from build123d import *

# Parameters (mm, degrees)
ESQUISSE2_W             = 17
ESQUISSE2_H             = 22
BASE_DEPTH              = 42
ESQUISSE3_R             = 6
VIDE_CERCLE_DEPTH       = 2
ESQUISSE4_R             = 1
AXE_ROUE_DEPTH          = 8
ESQUISSE6_R             = 1.5
COTE_DEPTH              = 4
ESQUISSE7_W             = 10.5
ESQUISSE7_H             = 8
AJUSTE_COTE_DEPTH       = 4
ESQUISSE8_W             = 7
ESQUISSE8_H             = 1
BLOC_MOTEUR_DEPTH       = 31
VODE_START              = -15
VODE_MOTEUR_DEPTH       = 15
ESQUISSE11_R            = 1
SORTIE_AXE_MOTEUR_DEPTH = 1
VIS_MOTEUR_1_DEPTH      = 6
VIS_MOTEUR_2_DEPTH      = 2
ESQUISSE15_R            = 1
VIS_MOTEUR_3_DEPTH      = 1


with BuildPart() as part:
    # Esquisse2 → Base (new body)
    with BuildSketch(Plane(origin=(0, 0, 0), x_dir=(1, 0, 0), z_dir=(0, 1, 0))):
        with Locations((-30.697167752, 0)):
            Rectangle(ESQUISSE2_W, ESQUISSE2_H)
    extrude(amount=-BASE_DEPTH)

    # Esquisse3 → VIDE CERCLE (cut)
    with BuildSketch(Plane.ZY.offset(39.197167752)):
        with Locations((0, -8.724551396)):
            Circle(ESQUISSE3_R)
        with Locations(Location((0, -33.275448604, 0), (0, 0, 180))):
            Circle(ESQUISSE3_R)
    extrude(amount=-VIDE_CERCLE_DEPTH, mode=Mode.SUBTRACT)

    # Esquisse4 → AXE ROUE (add)
    with BuildSketch(Plane.ZY.offset(37.197167752)):
        with BuildLine():
            Line((1.785357107, -6.974551396), (-1.785357107, -6.974551396))
            ThreePointArc((-1.785357107, -6.974551396), (-2.5, -8.724551396), (-1.785357107, -10.474551396))
            Line((-1.785357107, -10.474551396), (1.785357107, -10.474551396))
            ThreePointArc((1.785357107, -10.474551396), (2.5, -8.724551396), (1.785357107, -6.974551396))
        make_face()
        with Locations((0, -8.724551396)):
            Circle(ESQUISSE4_R, mode=Mode.SUBTRACT)
    extrude(amount=AXE_ROUE_DEPTH)

    # Esquisse6 → COTE (add)
    with BuildSketch(Plane.XY.offset(11)):
        with BuildLine():
            Line((-19.697167752, -2), (-16.197167752, -2))
            ThreePointArc((-16.197167752, -2), (-15.490060971, -2.292893219), (-15.197167752, -3))
            Line((-15.197167752, -3), (-15.197167752, -9))
            ThreePointArc((-15.197167752, -9), (-15.490060971, -9.707106781), (-16.197167752, -10))
            Line((-16.197167752, -10), (-19.697167752, -10))
            ThreePointArc((-19.697167752, -10), (-20.395192088, -10.520394841), (-21.197167752, -10.859339966))
            Line((-21.197167752, -10.859339966), (-21.197167752, -42))
            Line((-21.197167752, -42), (-22.197167752, -42))
            Line((-22.197167752, -42), (-22.197167752, -49))
            ThreePointArc((-22.197167752, -49), (-22.490060971, -49.707106781), (-23.197167752, -50))
            Line((-23.197167752, -50), (-31.697167752, -50))
            ThreePointArc((-31.697167752, -50), (-32.404274533, -49.707106781), (-32.697167752, -49))
            Line((-32.697167752, -49), (-32.697167752, -42))
            Line((-32.697167752, -42), (-39.197167752, -42))
            Line((-39.197167752, -42), (-39.197167752, 0))
            Line((-39.197167752, 0), (-22.197167752, 0))
            Line((-22.197167752, 0), (-21.197167752, 0))
            Line((-21.197167752, 0), (-21.197167752, -1.140660034))
            ThreePointArc((-21.197167752, -1.140660034), (-20.395192088, -1.479605159), (-19.697167752, -2))
        make_face()
        with Locations((-19.697167752, -6)):
            Circle(ESQUISSE6_R, mode=Mode.SUBTRACT)
        with Locations((-28.697167752, -35)):
            Circle(ESQUISSE6_R, mode=Mode.SUBTRACT)
        with Locations((-28.697167752, -45)):
            Circle(ESQUISSE6_R, mode=Mode.SUBTRACT)
    cote = extrude(amount=COTE_DEPTH)

    # SYM COTE: COTE across plane
    add(cote.mirror(Plane.XY))

    # Esquisse7 → AJUSTE COTE (cut)
    with BuildSketch(Plane.XY.offset(-11)):
        with Locations((-27.447167752, -46)):
            Rectangle(ESQUISSE7_W, ESQUISSE7_H)
    extrude(amount=-AJUSTE_COTE_DEPTH, mode=Mode.SUBTRACT)

    # Esquisse8 → BLOC MOTEUR (add)
    with BuildSketch(Plane(origin=(-22.197167752, 0, 0), x_dir=(0, 0, -1), z_dir=(1, 0, 0))):
        with BuildLine():
            ThreePointArc((-5.878988008, -24), (-10.75, -33), (-5.878988008, -42))
            Line((-5.878988008, -42), (-3.5, -42))
            Line((-3.5, -42), (3.5, -42))
            Line((3.5, -42), (5.878988008, -42))
            ThreePointArc((5.878988008, -42), (10.75, -33), (5.878988008, -24))
            Line((5.878988008, -24), (3.5, -24))
            Line((3.5, -24), (-3.5, -24))
            Line((-3.5, -24), (-5.878988008, -24))
        make_face()
        with Locations((0, -42.5)):
            Rectangle(ESQUISSE8_W, ESQUISSE8_H)
        with Locations((0, -23.5)):
            Rectangle(ESQUISSE8_W, ESQUISSE8_H)
    extrude(amount=BLOC_MOTEUR_DEPTH)

    # Esquisse10 → VODE MOTEUR (cut)
    with BuildSketch(Plane(origin=(8.802832248, 0, 0), x_dir=(0, 0, -1), z_dir=(1, 0, 0)).offset(VODE_START)):
        with BuildLine():
            Line((-5.878988008, -24), (-3.5, -24))
            Line((-3.5, -24), (-3.5, -25))
            Line((-3.5, -25), (-5.573374202, -25))
            ThreePointArc((-5.573374202, -25), (-9.75, -33), (-5.573374202, -41))
            Line((-5.573374202, -41), (-3.5, -41))
            Line((-3.5, -41), (-3.5, -42))
            Line((-3.5, -42), (-5.878988008, -42))
            ThreePointArc((-5.878988008, -42), (-10.75, -33), (-5.878988008, -24))
        make_face()
        with BuildLine():
            Line((3.5, -24), (5.878988008, -24))
            ThreePointArc((5.878988008, -24), (10.75, -33), (5.878988008, -42))
            Line((5.878988008, -42), (3.5, -42))
            Line((3.5, -42), (3.5, -41))
            Line((3.5, -41), (5.573374202, -41))
            ThreePointArc((5.573374202, -41), (9.75, -33), (5.573374202, -25))
            Line((5.573374202, -25), (3.5, -25))
            Line((3.5, -25), (3.5, -24))
        make_face()
    extrude(amount=VODE_MOTEUR_DEPTH, mode=Mode.SUBTRACT)

    # Esquisse11 → SORTIE AXE MOTEUR (add)
    with BuildSketch(Plane(origin=(8.802832248, 0, 0), x_dir=(0, 0, -1), z_dir=(1, 0, 0))):
        with Locations((0, -33)):
            Circle(ESQUISSE11_R)
    extrude(amount=SORTIE_AXE_MOTEUR_DEPTH)

    # Esquisse12 → VIS MOTEUR 1 (add)
    with BuildSketch(Plane(origin=(-22.197167752, 0, 0), x_dir=(0, 0, -1), z_dir=(1, 0, 0))):
        with BuildLine():
            Line((-2, -20.5), (-2, -23))
            Line((-2, -23), (2, -23))
            Line((2, -23), (2, -20.5))
            ThreePointArc((2, -20.5), (0, -18.5), (-2, -20.5))
        make_face()
        with BuildLine():
            Line((2, -45.5), (2, -43))
            Line((2, -43), (-2, -43))
            Line((-2, -43), (-2, -45.5))
            ThreePointArc((-2, -45.5), (0, -47.5), (2, -45.5))
        make_face()
    extrude(amount=VIS_MOTEUR_1_DEPTH)

    # Esquisse14 → VIS MOTEUR 2 (add)
    with BuildSketch(Plane(origin=(-16.197167752, 0, 0), x_dir=(0, 0, -1), z_dir=(1, 0, 0))):
        with BuildLine():
            Line((-2.5, -20.5), (-2.5, -23))
            Line((-2.5, -23), (2.5, -23))
            Line((2.5, -23), (2.5, -20.5))
            ThreePointArc((2.5, -20.5), (0, -18), (-2.5, -20.5))
        make_face()
        with BuildLine():
            Line((-2.5, -43), (2.5, -43))
            Line((2.5, -43), (2.5, -45.5))
            ThreePointArc((2.5, -45.5), (0, -48), (-2.5, -45.5))
            Line((-2.5, -45.5), (-2.5, -43))
        make_face()
    extrude(amount=VIS_MOTEUR_2_DEPTH)

    # Esquisse15 → VIS MOTEUR 3 (add)
    with BuildSketch(Plane(origin=(-14.197167752, 0, 0), x_dir=(0, 0, -1), z_dir=(1, 0, 0))):
        with Locations((0, -20.5)):
            Circle(ESQUISSE15_R)
        with Locations(Location((0, -45.5, 0), (0, 0, 180))):
            Circle(ESQUISSE15_R)
    extrude(amount=VIS_MOTEUR_3_DEPTH)


solid = part.part
Source: CAD feature listing. Evaluate the final solid. Frame: model axes, mm. A direction names the side the tool comes from. Coordinates: 2 decimals unless noted, no trailing zeros. Loops run counter-clockwise (first coordinate to the right, second up) from the corner with the lowest first, then second, coordinate; pieces in that order, holes last. Notation, with made-up numbers: (61, 69.5) - (67, 69.5) arc R30 ccw to (67, 101.5) - close; hole circle Ø11 at (-3.5, -22.5). An arc over 180 degrees is marked (long way). One line per question, with ' | ' between items.
1) Set-up query: faces 1 (the face through (-22.197, -44, 0)), 2 (the face through (-21.197, -26, -13)), 3 (the face through (-37.197, -9, 0)), 4 (the face through (-29, -35, 11)), 5 (the face through (9, -32, 0)). Return all of +Z, -Z, +X, -X, +Y, -Y with unobstructed straight access to the full face (end or side cutting, diameter ignored); none if empty.
Report:
face 1: -Z, -X, -Y | face 2: -Z, +X, -Y | face 3: -X | face 4: +Z | face 5: +X
2) Section B-B, the plane y = -6. Return loops of the section in (x, z).
Report:
outline: (-39.2, -15) - (-21.2, -15) - (-21.2, -11) - (-22.2, -11) - (-22.2, 11) - (-21.2, 11) - (-21.2, 15) - (-39.2, 15) - (-39.2, 5.35) - (-37.2, 5.35) - (-37.2, -5.35) - (-39.2, -5.35) - close; (-18.2, -15) - (-15.2, -15) - (-15.2, -11) - (-18.2, -11) - close; (-18.2, 11) - (-15.2, 11) - (-15.2, 15) - (-18.2, 15) - close
3) Section A-A, the plane z = 12.25. Return loops of the section in (x, y) (3 decimals), then the cut area to 3 significant figures.
Report:
outline: (-39.197, -42) - (-32.697, -42) - (-32.697, -49) arc R1 ccw to (-31.697, -50) - (-23.197, -50) arc R1 ccw to (-22.197, -49) - (-22.197, -42) - (-21.197, -42) - (-21.197, -10.859) arc R3.625 ccw to (-19.697, -10) - (-16.197, -10) arc R1 ccw to (-15.197, -9) - (-15.197, -3) arc R1 ccw to (-16.197, -2) - (-19.697, -2) arc R3.625 ccw to (-21.197, -1.141) - (-21.197, 0) - (-39.197, 0) - close; hole circle Ø3 at (-28.697, -45); hole circle Ø3 at (-28.697, -35); hole circle Ø3 at (-19.697, -6) | area: 867 mm²
4) Section C-C, the plane x = 6.5. Return loops of the section in (y, z).
Report:
outline: (-43, -3.5) - (-41, -3.5) - (-41, -5.57) arc R9.75 ccw to (-25, -5.57) - (-25, -3.5) - (-23, -3.5) - (-23, 3.5) - (-25, 3.5) - (-25, 5.57) arc R9.75 ccw to (-41, 5.57) - (-41, 3.5) - (-43, 3.5) - close
5) Line query: line 1 along Y through (x, z) = (-38.05, 0); line 2 along Y through (x, z) = (-20, -5); line 3 along Y through (x, z) = (-25.5, -11). Output: solid intervals per line, ascending.
Report:
line 1: y = -42 to -39.28, -27.28 to -14.72, -10.47 to -9.72, -7.72 to -6.97, -2.72 to 0 | line 2: y = -42 to -24 | line 3: y = -42 to 0
6) Section D-D, the plane y = -16. Return loops of the section in (x, z).
Report:
outline: (-39.2, -15) - (-21.2, -15) - (-21.2, -11) - (-22.2, -11) - (-22.2, 11) - (-21.2, 11) - (-21.2, 15) - (-39.2, 15) - close
7) First-contact query: P1, Ø3, axis at x = -21, z = -2, coming from the -Y side; P2, Ø1.2, axis at y = -7.5, z = -12.5, coming from the +X side; P3, Ø5, axis at x = -17.5, y = -38, coming from the -Z side. Flat tips, straight axial feed; report the tip coordinate or a pass-through.
Report:
P1: stops at y = -47.44 | P2: stops at x = -15.2 | P3: stops at z = -10.46
8) Pull-direction query (Y, two-part tool) for faces 6 (the face through (-15, -22, 2.5)), 7 (the face through (-37.197, -9, 3)), 8 (the face through (-20.41, -1.47, 12.97)); classes: released by +Y, released by -Y, zero draft, split by the parting line, or undercut.
Report:
face 6: zero draft | face 7: undercut | face 8: released by +Y
